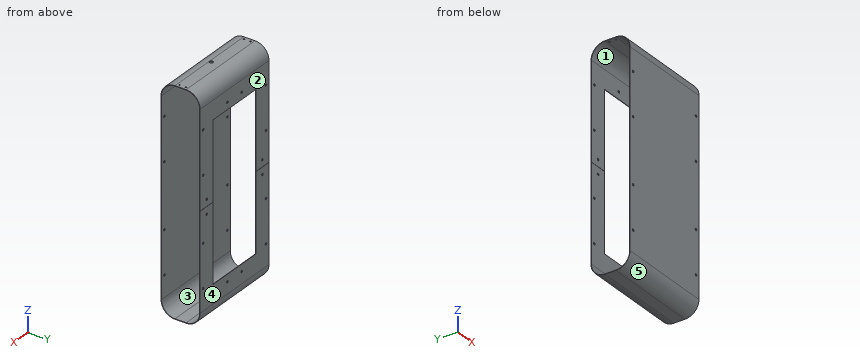
from build123d import *

# Parameters (mm, degrees)
SALIENTE_EXTRUIR1_DEPTH = 110
VACIADO2_T              = -1
CORTAR_EXTRUIR1_START   = -10
CORTAR_EXTRUIR1_DEPTH   = 10
CROQUIS8_R              = 1.5
CORTAR_EXTRUIR4_DEPTH   = 5
CROQUIS9_R              = 4
CORTAR_EXTRUIR5_DEPTH   = 5
CROQUIS10_R             = 2.5
CORTAR_EXTRUIR6_DEPTH   = 275.454003432
CROQUIS11_W             = 130
CROQUIS11_H             = 334
CORTAR_EXTRUIR7_DEPTH   = 8
CROQUIS12_R             = 2.5
CORTAR_EXTRUIR8_DEPTH   = 8
CROQUIS13_W             = 40
CROQUIS13_H             = 0.5
CORTAR_EXTRUIR9_DEPTH   = 1
CROQUIS14_R             = 2.5
CORTAR_EXTRUIR10_DEPTH  = 1


with BuildPart() as part:
    # Croquis1 → Saliente-Extruir1 (new, symmetric)
    with BuildSketch(Plane(origin=(0, 0, 0), x_dir=(0, 0, -1), z_dir=(1, 0, 0))):
        with BuildLine():
            Line((207, -42), (-207, -42))
            ThreePointArc((-207, -42), (-228.213203436, -33.213203436), (-237, -12))
            Line((-237, -12), (-237, 12))
            ThreePointArc((-237, 12), (-228.213203436, 33.213203436), (-207, 42))
            Line((-207, 42), (207, 42))
            ThreePointArc((207, 42), (228.213203436, 33.213203436), (237, 12))
            Line((237, 12), (237, -12))
            ThreePointArc((237, -12), (228.213203436, -33.213203436), (207, -42))
        make_face()
    extrude(amount=SALIENTE_EXTRUIR1_DEPTH, both=True)

    # Vaciado2
    vaciado2_openings = [part.faces().sort_by_distance(p)[0] for p in [
        (110, 0, 0),
    ]]
    offset(amount=VACIADO2_T, openings=vaciado2_openings, kind=Kind.INTERSECTION)

    # Croquis6 → Cortar-Extruir1 (cut)
    with BuildSketch(Plane.ZY.offset(110).offset(CORTAR_EXTRUIR1_START)):
        with BuildLine():
            Line((207, 42), (-207, 42))
            ThreePointArc((-207, 42), (-228.213203436, 33.213203436), (-237, 12))
            Line((-237, 12), (-237, -12))
            ThreePointArc((-237, -12), (-228.213203436, -33.213203436), (-207, -42))
            Line((-207, -42), (207, -42))
            ThreePointArc((207, -42), (228.213203436, -33.213203436), (237, -12))
            Line((237, -12), (237, 12))
            ThreePointArc((237, 12), (228.213203436, 33.213203436), (207, 42))
        make_face()
    extrude(amount=CORTAR_EXTRUIR1_DEPTH, mode=Mode.SUBTRACT)

    # Croquis8 → Cortar-Extruir4 (cut)
    with BuildSketch(Plane.XY.offset(237)):
        with Locations((103.5, 7)):
            Circle(CROQUIS8_R)
        with Locations((103.5, -7)):
            Circle(CROQUIS8_R)
        with Locations(Location((-93.5, -7, 0), (0, 0, 90))):
            Circle(CROQUIS8_R)
        with Locations(Location((-93.5, 7, 0), (0, 0, 90))):
            Circle(CROQUIS8_R)
    extrude(amount=-CORTAR_EXTRUIR4_DEPTH, mode=Mode.SUBTRACT)

    # Croquis9 → Cortar-Extruir5 (cut)
    with BuildSketch(Plane.XY.offset(237)):
        with Locations(Location((5, -8, 0), (0, 0, 270))):
            Circle(CROQUIS9_R)
    extrude(amount=-CORTAR_EXTRUIR5_DEPTH, mode=Mode.SUBTRACT)

    # Croquis10 → Cortar-Extruir6 (cut, through all)
    with BuildSketch(Plane(origin=(0, 42, 0), x_dir=(1, 0, 0), z_dir=(0, 1, 0))):
        with Locations(Location((101, 161.01, 0), (0, 0, 270))):
            Circle(CROQUIS10_R)
        with Locations(Location((101, 69.01, 0), (0, 0, 270))):
            Circle(CROQUIS10_R)
        with Locations(Location((-91, 69.01, 0), (0, 0, 270))):
            Circle(CROQUIS10_R)
        with Locations(Location((-91, 161.01, 0), (0, 0, 270))):
            Circle(CROQUIS10_R)
        with Locations(Location((101, -69.01, 0), (0, 0, 270))):
            Circle(CROQUIS10_R)
        with Locations(Location((101, -161.01, 0), (0, 0, 270))):
            Circle(CROQUIS10_R)
        with Locations(Location((-91, -161.01, 0), (0, 0, 270))):
            Circle(CROQUIS10_R)
        with Locations(Location((-91, -69.01, 0), (0, 0, 270))):
            Circle(CROQUIS10_R)
    extrude(amount=-CORTAR_EXTRUIR6_DEPTH, mode=Mode.SUBTRACT)

    # Croquis11 → Cortar-Extruir7 (cut)
    with BuildSketch(Plane(origin=(0, 42, 0), x_dir=(1, 0, 0), z_dir=(0, 1, 0))):
        with Locations((5, 0)):
            Rectangle(CROQUIS11_W, CROQUIS11_H)
    extrude(amount=-CORTAR_EXTRUIR7_DEPTH, mode=Mode.SUBTRACT)

    # Croquis12 → Cortar-Extruir8 (cut)
    with BuildSketch(Plane(origin=(0, 42, 0), x_dir=(1, 0, 0), z_dir=(0, 1, 0))):
        with Locations(Location((-16.666666667, 182, 0), (0, 0, 270))):
            Circle(CROQUIS12_R)
        with Locations(Location((26.666666667, 182, 0), (0, 0, 270))):
            Circle(CROQUIS12_R)
        with Locations(Location((26.666666667, -182, 0), (0, 0, 90))):
            Circle(CROQUIS12_R)
        with Locations(Location((-16.666666667, -182, 0), (0, 0, 90))):
            Circle(CROQUIS12_R)
    extrude(amount=-CORTAR_EXTRUIR8_DEPTH, mode=Mode.SUBTRACT)

    # Croquis13 → Cortar-Extruir9 (cut)
    with BuildSketch(Plane(origin=(0, 42, 0), x_dir=(1, 0, 0), z_dir=(0, 1, 0))):
        with Locations((-80, -0.25)):
            Rectangle(CROQUIS13_W, CROQUIS13_H)
        with Locations((90, -0.25)):
            Rectangle(CROQUIS13_W, CROQUIS13_H)
    extrude(amount=-CORTAR_EXTRUIR9_DEPTH, mode=Mode.SUBTRACT)

    # Croquis14 → Cortar-Extruir10 (cut)
    with BuildSketch(Plane(origin=(0, 42, 0), x_dir=(1, 0, 0), z_dir=(0, 1, 0))):
        with Locations(Location((90, 15, 0), (0, 0, 270))):
            Circle(CROQUIS14_R)
        with Locations(Location((90, -15, 0), (0, 0, 270))):
            Circle(CROQUIS14_R)
        with Locations(Location((-80, -15, 0), (0, 0, 90))):
            Circle(CROQUIS14_R)
        with Locations(Location((-80, 15, 0), (0, 0, 90))):
            Circle(CROQUIS14_R)
    extrude(amount=-CORTAR_EXTRUIR10_DEPTH, mode=Mode.SUBTRACT)


solid = part.part
Here's how the part is built. I have some questions about the finished solid (model axes, mm). Face numbers are marked on the shaded views. A direction names the side the tool comes from. Round coordinates to 2 decimals unless told otherwise and drop trailing zeros. Loops run counter-clockwise (first coordinate to the right, second up) from the corner with the lowest first, then second, coordinate; pieces in that order, holes last. Notation, with made-up numbers: (20.5, 18) - (68.5, 18) arc R22 ccw to (68.5, 44) - close; hole circle Ø8 at (-22.5, 54.5). An arc over 180 degrees is marked (long way). One line per question, with ' | ' between items. Start each with the question number.
Q1. I want a section at D-D (y = -32.5). Write out the boundary of the cut face in (x, z).
Q2. Please list where these lines run through material, in increasing order: line 1 (X direction, y = 41.45, z = 69.01); line 2 (X direction, y = -41.4, z = -161.01); line 3 (Z direction, x = 42.5, y = 0). Write a range as [from, to].
Q3. For the marked faces 1 and 2, which set-ups out of +Z, -Z, +X, -X, +Y, -Y let a thin tool reach every point of the face, with its end or its side?
Q4. Will these pins go through, and if not, where does the flat tip stop? pin 1 (2 mm diameter, centred on x = 55, z = -83.5, fed in from +Y); pin 2 (4 mm diameter, centred on x = 77, y = -18, fed in from -Z).
Q5. We'd pull the mould along Y, two halves only. Please class the marked faces 3, 4 and 5: +Y half, -Y half, draft (parallel to the pull), parting line (faces both ways), or undercut.
Q6. I want a section at A-A (z = -8). Write out the boundary of the cut face in (x, y).
Q7. I want a section at B-B (y = 33.5). Write out the boundary of the cut face in (x, z).
Q8. I want a section at C-C (x = -69). Write out the boundary of the cut face in (y, z).
Response values:
1) outline: (-100, -228.9) - (110, -228.9) - (110, -227.51) - (-100, -227.51) - close; (-100, 227.51) - (110, 227.51) - (110, 228.9) - (-100, 228.9) - close
2) line 1: x = [-100, -93.5], [-88.5, -60], [70, 98.5], [103.5, 110] | line 2: x = [-100, -93.5], [-88.5, 98.5], [103.5, 110] | line 3: z = [-237, -236], [236, 237]
3) face 1: +X, -X | face 2: +Z, -Z, +X, -X, +Y
4) pin 1: stops at y = -41 | pin 2: stops at z = -236.73
5) face 3: undercut | face 4: +Y half | face 5: -Y half
6) outline: (-100, -42) - (110, -42) - (110, -41) - (-100, -41) - close; (-100, 41) - (-60, 41) - (-60, 42) - (-100, 42) - close; (70, 41) - (110, 41) - (110, 42) - (70, 42) - close
7) outline: (-100, -227.92) - (110, -227.92) - (110, -226.46) - (-100, -226.46) - close; (-100, 226.46) - (110, 226.46) - (110, 227.92) - (-100, 227.92) - close
8) outline: (-42, -207) arc R30 ccw to (-12, -237) - (12, -237) arc R30 ccw to (42, -207) - (42, 0) - (41, 0) - (41, -207) arc R29 cw to (12, -236) - (-12, -236) arc R29 cw to (-41, -207) - (-41, 207) arc R29 cw to (-12, 236) - (12, 236) arc R29 cw to (41, 207) - (41, 0.5) - (42, 0.5) - (42, 207) arc R30 ccw to (12, 237) - (-12, 237) arc R30 ccw to (-42, 207) - close
